```python
from build123d import *

# Parameters (mm, degrees)
CUT_EXTRUDE1_DEPTH = 2.5


with BuildPart() as part:
    # Sketch3 → Revolve1 (revolve)
    with BuildSketch(Plane(origin=(0, 0, 0), x_dir=(0, 0, -1), z_dir=(1, 0, 0)), mode=Mode.PRIVATE) as revolve1_sk:
        with BuildLine():
            Line((-7.5, 3.874791847), (-7.5, 2))
            Line((-7.5, 2), (-5, 2))
            Line((-5, 2), (-5, 0))
            Line((-5, 0), (7.5, 0))
            Line((7.5, 0), (7.5, 1.980384758))
            Line((7.5, 1.980384758), (6.980384758, 2.5))
            Line((6.980384758, 2.5), (-2.5, 2.5))
            Line((-2.5, 2.5), (-2.5, 3.874791847))
            ThreePointArc((-2.5, 3.874791847), (-2.50647024, 3.907319939), (-2.524895924, 3.934895924))
            Line((-2.524895924, 3.934895924), (-2.815104076, 4.225104076))
            ThreePointArc((-2.815104076, 4.225104076), (-2.842680061, 4.24352976), (-2.875208153, 4.25))
            Line((-2.875208153, 4.25), (-7.124791847, 4.25))
            ThreePointArc((-7.124791847, 4.25), (-7.157319939, 4.24352976), (-7.184895924, 4.225104076))
            Line((-7.184895924, 4.225104076), (-7.475104076, 3.934895924))
            ThreePointArc((-7.475104076, 3.934895924), (-7.49352976, 3.907319939), (-7.5, 3.874791847))
        make_face()
    revolve(revolve1_sk.sketch.rotate(Axis((0, 0, 7.5), (0, 0, -1)), 90), axis=Axis((0, 0, 7.5), (0, 0, -1)))

    # Sketch4 → Cut-Extrude1 (cut)
    with BuildSketch(Plane.XY.offset(7.5)):
        Polygon((0, 2.309401077), (-2, 1.154700538), (-2, -1.154700538), (0, -2.309401077), (2, -1.154700538), (2, 1.154700538), align=None)
    extrude(amount=-CUT_EXTRUDE1_DEPTH, mode=Mode.SUBTRACT)

    # Cut-Extrude2 cone 1 section (through the dimple's axis) → Cut-Extrude2 (revolve, cut)
    with BuildSketch(Plane(origin=(0, 0, 7.5), x_dir=(0, -1, 0), z_dir=(1, 0, 0))):
        Polygon((0, 0), (2.309401077, 0), (0, 2.309401077), align=None)
    revolve(axis=Axis((0, 0, 7.5), (0, 0, -1)), mode=Mode.SUBTRACT)

    # Cut-Extrude3 cone 1 section (through the dimple's axis) → Cut-Extrude3 (revolve, cut)
    with BuildSketch(Plane(origin=(0, 0, 5), x_dir=(0, -1, 0), z_dir=(1, 0, 0))):
        Polygon((0, 0), (2, 0), (0, 1.154700538), align=None)
    revolve(axis=Axis((0, 0, 5), (0, 0, -1)), mode=Mode.SUBTRACT)


solid = part.part
```
The listing builds one solid part. Answer for the finished solid, in the listing's coordinates (mm). Round coordinates to 2 decimals unless told otherwise and drop trailing zeros. Loops run counter-clockwise (first coordinate to the right, second up) from the corner with the lowest first, then second, coordinate; pieces in that order, holes last. Notation, with made-up numbers: (62, -26.5) - (93, -26.5) arc R11 ccw to (93, -21.5) - close; hole circle Ø4 at (39, -27). An arc over 180 degrees is marked (long way). Use one line per item in the form item = value. Start each with the question number.
1. For a pull along X with two mould halves and no side action, classify faces 1 (the face through (2, 2, 7.5)), 2 (the face through (-0.553, -4.214, 5.03)), 3 (the face through (0.99, -1.74, 6.27)) as pulls with the +X half, pulls with the -X half, needs draft (parallel to the pull), parting line crosses it, or undercut.
2. Consider line 1 (Z direction, x = -0.75, y = 2.5); line 2 (Y direction, x = 1.5, z = 1.25); line 3 (X direction, y = 2, z = 7). Determine where each line is inside the solid, lowest interval first. Write a range as [from, to].
3. The part is cut by section A-A on z = -2.5. Determine the outline of the cut face in (x, y), then the cut area to 3 significant figures.
4. The part is cut by section B-B on z = 4.75. Determine the outline of the cut face in (x, y).
5. Given pin 1 Ø5 at (y, z) = (2, -3.5) entering from -X; pin 2 Ø4 at (x, z) = (-3, 3.5) entering from -Y; pin 3 Ø1.1 at (x, y) = (1.5, -0.5) entering from +Z, each flat-ended and moving along its own axis, determine where each tip first touches the part or whether it passes through.
Geometry check:
q1.face_1 = needs draft
q1.face_2 = parting line crosses it
q1.face_3 = undercut
q2.line_1 = [2.5, 7.5]
q2.line_2 = [-2, 2]
q2.line_3 = [-3.75, -0.54], [0.54, 3.75]
q3.outline = circle Ø5 at (0, 0)
q3.area = 19.6 mm^2
q4.outline = circle Ø8.5 at (0, 0); hole circle Ø3.13 at (0, 0)
q5.pin_1 = -2.5
q5.pin_2 = -4.13
q5.pin_3 = 7.32
